Input: part model. Units: mm. Frame: model coordinates. A direction names the side the tool comes from. Give positions to 0.01 mm unless a question says otherwise; leave off trailing zeros. Order: outer loops, then holes, each group sorted by start corner. A loop starts at its lowest first (then second) coordinate and runs counter-clockwise, first axis right, second up. Notation, with made-up numbers: (73, 83.5) - (131, 83.5) arc R9 ccw to (131, 94.5) - close; hole circle Ø6 at (-9, 6). An arc over 180 degrees is marked (long way). Use a Markdown table: item, result.
from build123d import *

# Parameters (mm, degrees)
SKETCH3_R           = 8
BOSS_EXTRUDE3_DEPTH = 5
CUT_EXTRUDE1_DEPTH  = 6
SKETCH5_W           = 6.35
SKETCH5_H           = 6.35
CUT_EXTRUDE2_DEPTH  = 6


with BuildPart() as part:
    # Sketch3 → Boss-Extrude3 (new body)
    with BuildSketch(Plane(origin=(0, 0, 0), x_dir=(1, 0, 0), z_dir=(0, 1, 0))):
        Circle(SKETCH3_R)
    extrude(amount=BOSS_EXTRUDE3_DEPTH)

    # Sketch4 → Cut-Extrude1 (cut, through all)
    with BuildSketch(Plane(origin=(0, 5, 0), x_dir=(1, 0, 0), z_dir=(0, 1, 0))):
        with BuildLine():
            Line((-0.6, 6), (0.6, 6))
            ThreePointArc((0.6, 6), (0.851894231, 6.997970737), (1.383186803, 7.879517388))
            ThreePointArc((1.383186803, 7.879517388), (0, 8), (-1.383186803, 7.879517388))
            ThreePointArc((-1.383186803, 7.879517388), (-0.851894231, 6.997970737), (-0.6, 6))
        make_face()
        with BuildLine():
            Line((2.062721114, 5.666143451), (3.143883755, 5.145482964))
            ThreePointArc((3.143883755, 5.145482964), (3.80383589, 5.935330718), (4.665002715, 6.499057599))
            ThreePointArc((4.665002715, 6.499057599), (3.471069913, 7.207750943), (2.172586219, 7.699342123))
            ThreePointArc((2.172586219, 7.699342123), (2.268775529, 6.674576827), (2.062721114, 5.666143451))
        make_face()
        with BuildLine():
            Line((4.316895014, 4.210037701), (5.065082776, 3.271839922))
            ThreePointArc((5.065082776, 3.271839922), (6.002381201, 3.697125659), (7.022857626, 3.831379746))
            ThreePointArc((7.022857626, 3.831379746), (6.25465186, 4.987918415), (5.298051895, 5.994217724))
            ThreePointArc((5.298051895, 5.994217724), (4.94008647, 5.029201118), (4.316895014, 4.210037701))
        make_face()
        with BuildLine():
            Line((5.716054913, 1.920082351), (5.983080033, 0.750168856))
            ThreePointArc((5.983080033, 0.750168856), (7.0120813, 0.72665952), (7.989749455, 0.404850146))
            ThreePointArc((7.989749455, 0.404850146), (7.799423297, 1.780167472), (7.374173417, 3.10186499))
            ThreePointArc((7.374173417, 3.10186499), (6.6329527, 2.387730448), (5.716054913, 1.920082351))
        make_face()
        with BuildLine():
            Line((5.983080033, -0.750168856), (5.716054913, -1.920082351))
            ThreePointArc((5.716054913, -1.920082351), (6.6329527, -2.387730448), (7.374173417, -3.10186499))
            ThreePointArc((7.374173417, -3.10186499), (7.799423297, -1.780167472), (7.989749455, -0.404850146))
            ThreePointArc((7.989749455, -0.404850146), (7.0120813, -0.72665952), (5.983080033, -0.750168856))
        make_face()
        with BuildLine():
            Line((5.065082776, -3.271839922), (4.316895014, -4.210037701))
            ThreePointArc((4.316895014, -4.210037701), (4.94008647, -5.029201118), (5.298051895, -5.994217724))
            ThreePointArc((5.298051895, -5.994217724), (6.25465186, -4.987918415), (7.022857626, -3.831379746))
            ThreePointArc((7.022857626, -3.831379746), (6.002381201, -3.697125659), (5.065082776, -3.271839922))
        make_face()
        with BuildLine():
            Line((3.143883755, -5.145482964), (2.062721114, -5.666143451))
            ThreePointArc((2.062721114, -5.666143451), (2.268775529, -6.674576827), (2.172586219, -7.699342123))
            ThreePointArc((2.172586219, -7.699342123), (3.471069913, -7.207750943), (4.665002715, -6.499057599))
            ThreePointArc((4.665002715, -6.499057599), (3.80383589, -5.935330718), (3.143883755, -5.145482964))
        make_face()
        with BuildLine():
            Line((0.6, -6), (-0.6, -6))
            ThreePointArc((-0.6, -6), (-0.851894231, -6.997970737), (-1.383186803, -7.879517388))
            ThreePointArc((-1.383186803, -7.879517388), (0, -8), (1.383186803, -7.879517388))
            ThreePointArc((1.383186803, -7.879517388), (0.851894231, -6.997970737), (0.6, -6))
        make_face()
        with BuildLine():
            Line((-2.062721114, -5.666143451), (-3.143883755, -5.145482964))
            ThreePointArc((-3.143883755, -5.145482964), (-3.80383589, -5.935330718), (-4.665002715, -6.499057599))
            ThreePointArc((-4.665002715, -6.499057599), (-3.471069913, -7.207750943), (-2.172586219, -7.699342123))
            ThreePointArc((-2.172586219, -7.699342123), (-2.268775529, -6.674576827), (-2.062721114, -5.666143451))
        make_face()
        with BuildLine():
            Line((-4.316895014, -4.210037701), (-5.065082776, -3.271839922))
            ThreePointArc((-5.065082776, -3.271839922), (-6.002381201, -3.697125659), (-7.022857626, -3.831379746))
            ThreePointArc((-7.022857626, -3.831379746), (-6.25465186, -4.987918415), (-5.298051895, -5.994217724))
            ThreePointArc((-5.298051895, -5.994217724), (-4.94008647, -5.029201118), (-4.316895014, -4.210037701))
        make_face()
        with BuildLine():
            Line((-5.716054913, -1.920082351), (-5.983080033, -0.750168856))
            ThreePointArc((-5.983080033, -0.750168856), (-7.0120813, -0.72665952), (-7.989749455, -0.404850146))
            ThreePointArc((-7.989749455, -0.404850146), (-7.799423297, -1.780167472), (-7.374173417, -3.10186499))
            ThreePointArc((-7.374173417, -3.10186499), (-6.6329527, -2.387730448), (-5.716054913, -1.920082351))
        make_face()
        with BuildLine():
            Line((-5.983080033, 0.750168856), (-5.716054913, 1.920082351))
            ThreePointArc((-5.716054913, 1.920082351), (-6.6329527, 2.387730448), (-7.374173417, 3.10186499))
            ThreePointArc((-7.374173417, 3.10186499), (-7.799423297, 1.780167472), (-7.989749455, 0.404850146))
            ThreePointArc((-7.989749455, 0.404850146), (-7.0120813, 0.72665952), (-5.983080033, 0.750168856))
        make_face()
        with BuildLine():
            Line((-5.065082776, 3.271839922), (-4.316895014, 4.210037701))
            ThreePointArc((-4.316895014, 4.210037701), (-4.94008647, 5.029201118), (-5.298051895, 5.994217724))
            ThreePointArc((-5.298051895, 5.994217724), (-6.25465186, 4.987918415), (-7.022857626, 3.831379746))
            ThreePointArc((-7.022857626, 3.831379746), (-6.002381201, 3.697125659), (-5.065082776, 3.271839922))
        make_face()
        with BuildLine():
            Line((-3.143883755, 5.145482964), (-2.062721114, 5.666143451))
            ThreePointArc((-2.062721114, 5.666143451), (-2.268775529, 6.674576827), (-2.172586219, 7.699342123))
            ThreePointArc((-2.172586219, 7.699342123), (-3.471069913, 7.207750943), (-4.665002715, 6.499057599))
            ThreePointArc((-4.665002715, 6.499057599), (-3.80383589, 5.935330718), (-3.143883755, 5.145482964))
        make_face()
    extrude(amount=-CUT_EXTRUDE1_DEPTH, mode=Mode.SUBTRACT)

    # Sketch5 → Cut-Extrude2 (cut, through all)
    with BuildSketch(Plane(origin=(0, 5, 0), x_dir=(1, 0, 0), z_dir=(0, 1, 0))):
        Rectangle(SKETCH5_W, SKETCH5_H)
    extrude(amount=-CUT_EXTRUDE2_DEPTH, mode=Mode.SUBTRACT)


solid = part.part
1. Section query B-B (z = -6.25). Return loops of the section in (x, y).
Response:
| item | result |
|---|---|
| outline | (-4.99, 0) - (-4.22, 0) - (-4.22, 5) - (-4.99, 5) - close; (-2.22, 0) - (-0.63, 0) - (-0.63, 5) - (-2.22, 5) - close; (0.63, 0) - (2.22, 0) - (2.22, 5) - (0.63, 5) - close; (4.22, 0) - (4.99, 0) - (4.99, 5) - (4.22, 5) - close |
2. Section query C-C (x = -6.25). Return loops of the section in (y, z), then the cut area to 3 significant figures.
Response:
| item | result |
|---|---|
| outline | (0, -3.76) - (5, -3.76) - (5, -2.15) - (0, -2.15) - close; (0, -0.77) - (5, -0.77) - (5, 0.77) - (0, 0.77) - close; (0, 2.15) - (5, 2.15) - (5, 3.76) - (0, 3.76) - close |
| area | 23.8 mm^2 |
3. Material intervals for line 1 along Z through (x, y) = (6.75, 3.75); line 2 along Z through (x, y) = (-0.5, 4.4) (3 decimals); line 3 along Z through (x, y) = (7, 2.65), sorted ascending.
Response:
| item | result |
|---|---|
| line 1 | z = -3.83 to -2.47, -0.76 to 0.76, 2.47 to 3.83 |
| line 2 | z = -6 to -3.175, 3.175 to 6 |
| line 3 | z = -3.83 to -2.69, -0.73 to 0.73, 2.69 to 3.83 |
4. Pin query (flat end, axial travel): pin 1 (1.5 mm diameter, centred on y = 1.5, z = -1, fed in from -X); pin 2 (2 mm diameter, centred on y = 2.5, z = 4.5, fed in from -X). Return the tip coordinate at first contact, or that it passes through.
Response:
| item | result |
|---|---|
| pin 1 | stops at x = -8 |
| pin 2 | stops at x = -7.19 |
5. Section query A-A (x = -0.25). Return loops of the section in (y, z) (3 decimals), then the cut area to 4 significant figures.
Response:
| item | result |
|---|---|
| outline | (0, -6) - (5, -6) - (5, -3.175) - (0, -3.175) - close; (0, 3.175) - (5, 3.175) - (5, 6) - (0, 6) - close |
| area | 28.25 mm^2 |
6. Set-up query: faces 1 (the face through (-6.645, 2.535, 2.396)), 2 (the face through (-3.793, 2.535, 5.926)), 3 (the face through (4.686, 2.535, -3.748)). Return all of +Z, -Z, +X, -X, +Y, -Y with unobstructed straight access to the full face (end or side cutting, diameter ignored); none if empty.
Response:
| item | result |
|---|---|
| face 1 | -X, +Y, -Y |
| face 2 | +Z, +Y, -Y |
| face 3 | +Y, -Y |
